CAD build for the part. Positions are in the model's coordinates, mm. Face numbers are marked on the shaded views. Give positions to 0.01 mm unless a question says otherwise; leave off trailing zeros. Order: outer loops, then holes, each group sorted by start corner. A loop starts at its lowest first (then second) coordinate and runs counter-clockwise, first axis right, second up.
Item 1: Band-saw the part on A-A on x = 292. Give the cut face in (y, z), plus the area to 3 significant figures.
Item 2: Flat gauge pins, fed straight in: P1, Ø5, axis at x = 170.5, y = 45, coming from the -Z side; P2, Ø1.6, axis at x = 306.49, z = -84.02, coming from the +Y side. Where does each tip first touch, or does it go through?
Item 3: Band-saw the part on B-B on y = 118.5. Give the cut face in (x, z), plus the area to 3 significant figures.
Item 4: Wall check: L1, parallel to X at y = 2.9, z = -84.5; L2, parallel to Y at x = 137, z = -81; L3, parallel to X at y = 41, z = -86.75. Give the ranges that are in metal, low to high.
Item 5: Two-plate mould, pull along X, no slides. Class the marked faces 1 and 2: released by +X, released by -X, zero draft, split by the parting line, or undercut.
```python
from build123d import *

# Parameters (mm, degrees)
BOSS_EXTRUDE1_START = -80
SKETCH1_W           = 323.749339931
SKETCH1_H           = 127.712624425
BOSS_EXTRUDE1_DEPTH = 4
SKETCH4_W           = 323.749339931
SKETCH4_H           = 127.712624425
SKETCH4_W_2         = 315.749339931
SKETCH4_H_2         = 119.712624425
BOSS_EXTRUDE2_DEPTH = 15
SKETCH6_R           = 1.55
CUT_EXTRUDE2_DEPTH  = 6
SKETCH10_R          = 1.29987
CUT_EXTRUDE3_DEPTH  = 6
FILLET1_R           = 3


with BuildPart() as part:
    # Sketch1 → Boss-Extrude1 (new body)
    with BuildSketch(Plane.XY.offset(BOSS_EXTRUDE1_START)):
        with Locations((196.446669966, 63.856312213)):
            Rectangle(SKETCH1_W, SKETCH1_H)
    extrude(amount=BOSS_EXTRUDE1_DEPTH)

    # Sketch4 → Boss-Extrude2 (add)
    with BuildSketch(Plane.XY.offset(-76)):
        with Locations((196.446669966, 63.856312213)):
            Rectangle(SKETCH4_W, SKETCH4_H)
        with Locations((196.446669966, 63.856312213)):
            Rectangle(SKETCH4_W_2, SKETCH4_H_2, mode=Mode.SUBTRACT)
    extrude(amount=-BOSS_EXTRUDE2_DEPTH)

    # Sketch6 → Cut-Extrude2 (cut)
    with BuildSketch(Plane.XZ):
        with Locations(Location((207.946669965, -84.5, 0), (0, 0, 270))):
            Circle(SKETCH6_R)
        with Locations(Location((184.946669965, -84.5, 0), (0, 0, 270))):
            Circle(SKETCH6_R)
    extrude(amount=-CUT_EXTRUDE2_DEPTH, mode=Mode.SUBTRACT)

    # Sketch10 → Cut-Extrude3 (cut)
    with BuildSketch(Plane(origin=(0, 127.712624425, 0), x_dir=(1, 0, 0), z_dir=(0, 1, 0))):
        with Locations(Location((306.489689931, 84.015230538, 0), (0, 0, 270))):
            Circle(SKETCH10_R)
        with Locations(Location((318.821789931, 84.015230538, 0), (0, 0, 270))):
            Circle(SKETCH10_R)
        with Locations(Location((73.73825, 84.015230538, 0), (0, 0, 270))):
            Circle(SKETCH10_R)
        with Locations(Location((86.07035, 84.015230538, 0), (0, 0, 270))):
            Circle(SKETCH10_R)
    extrude(amount=-CUT_EXTRUDE3_DEPTH, mode=Mode.SUBTRACT)

    # Fillet1
    fillet1_edges = [part.edges().sort_by_distance(p)[0] for p in [
        (196.446669965, 127.712624425, -91),
    ]]
    fillet(fillet1_edges, radius=FILLET1_R)


solid = part.part
```
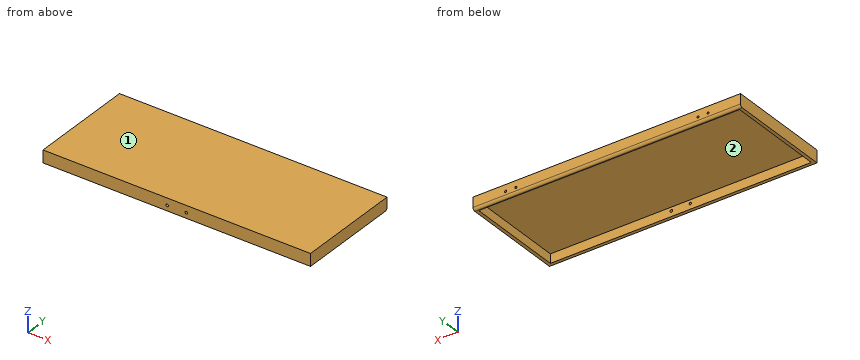
The answers:
1. outline: (0, -91) - (4, -91) - (4, -80) - (123.71, -80) - (123.71, -91) - (124.71, -91) arc R3 ccw to (127.71, -88) - (127.71, -76) - (0, -76) - close
1. area: 597 mm2
2. P1: stops at z = -80
2. P2: stops at y = 4
3. outline: (34.57, -91) - (38.57, -91) - (38.57, -80) - (354.32, -80) - (354.32, -91) - (358.32, -91) - (358.32, -76) - (34.57, -76) - close
3. area: 1,380 mm2
4. L1: x = 34.57 to 183.4, 186.5 to 206.4, 209.5 to 358.32
4. L2: y = 0 to 4, 123.71 to 127.71
4. L3: x = 34.57 to 38.57, 354.32 to 358.32
5. face 1: zero draft
5. face 2: undercut
